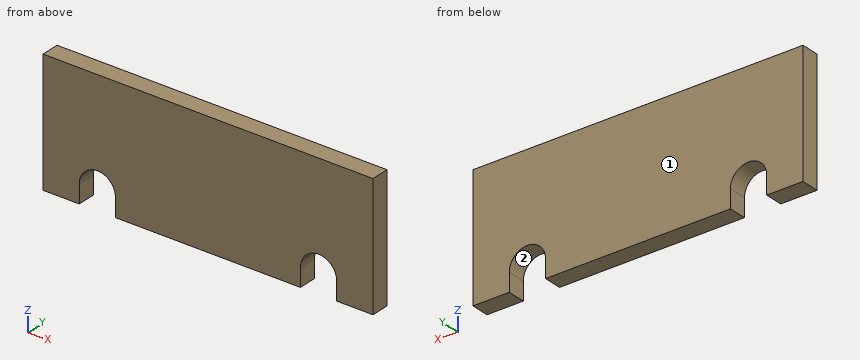
from build123d import *

# Parameters (mm, degrees)
SKETCH1_W           = 115.57
SKETCH1_H           = 43.18
BOSS_EXTRUDE1_DEPTH = 6.35
CUT_EXTRUDE1_DEPTH  = 7.35


with BuildPart() as part:
    # Sketch1 → Boss-Extrude1 (new body)
    with BuildSketch(Plane(origin=(0, 0, 0), x_dir=(1, 0, 0), z_dir=(0, 1, 0))):
        with Locations((57.785, 21.59)):
            Rectangle(SKETCH1_W, SKETCH1_H)
    extrude(amount=BOSS_EXTRUDE1_DEPTH)

    # Sketch2 → Cut-Extrude1 (cut, through all)
    with BuildSketch(Plane(origin=(0, 6.35, 0), x_dir=(1, 0, 0), z_dir=(0, 1, 0))):
        with BuildLine():
            Line((25.4, 52.705), (25.4, 36.83))
            ThreePointArc((25.4, 36.83), (19.05, 30.48), (12.7, 36.83))
            Line((12.7, 36.83), (12.7, 52.705))
            Line((12.7, 52.705), (25.4, 52.705))
        make_face()
        with BuildLine():
            Line((102.87, 52.705), (90.17, 52.705))
            Line((90.17, 52.705), (90.17, 36.83))
            ThreePointArc((90.17, 36.83), (96.52, 30.48), (102.87, 36.83))
            Line((102.87, 36.83), (102.87, 52.705))
        make_face()
    extrude(amount=-CUT_EXTRUDE1_DEPTH, mode=Mode.SUBTRACT)


solid = part.part
Source: CAD feature listing. Evaluate the final solid. Frame: model axes, mm. Face numbers are marked on the shaded views. Round coordinates to 2 decimals unless told otherwise and drop trailing zeros. Loops run counter-clockwise (first coordinate to the right, second up) from the corner with the lowest first, then second, coordinate; pieces in that order, holes last.
Q1. Mould query, pull axis X, two halves, no side actions, for the marked faces 1 and 2. Classes: pulls with the +X half, pulls with the -X half, needs draft (parallel to the pull), parting line crosses it, or undercut.
Q2. Ray query, line 1 (X direction, y = 0.5, z = -40.5); line 2 (X direction, y = 1.25, z = -35). Return the intervals inside material, ascending.
Q3. Section A-A, the plane z = -39. Return loops of the section in (x, y).
Q4. Section C-C, the plane x = 96.52. Return loops of the section in (y, z).
Q5. Section B-B, the plane y = 1.5. Return loops of the section in (x, z), plus the area to 3 significant figures.
Solutions:
1. face 1: needs draft
1. face 2: undercut
2. line 1: x = 0 to 12.7, 25.4 to 90.17, 102.87 to 115.57
2. line 2: x = 0 to 12.97, 25.13 to 90.44, 102.6 to 115.57
3. outline: (0, 0) - (12.7, 0) - (12.7, 6.35) - (0, 6.35) - close; (25.4, 0) - (90.17, 0) - (90.17, 6.35) - (25.4, 6.35) - close; (102.87, 0) - (115.57, 0) - (115.57, 6.35) - (102.87, 6.35) - close
4. outline: (0, -30.48) - (6.35, -30.48) - (6.35, 0) - (0, 0) - close
5. outline: (0, -43.18) - (12.7, -43.18) - (12.7, -36.83) arc R6.35 cw to (25.4, -36.83) - (25.4, -43.18) - (90.17, -43.18) - (90.17, -36.83) arc R6.35 cw to (102.87, -36.83) - (102.87, -43.18) - (115.57, -43.18) - (115.57, 0) - (0, 0) - close
5. area: 4,700 mm2
